Can you work these out from the model? Positions are in its coordinate system, mm. Face numbers are marked on the shaded views. A direction names the side the tool comes from. Give positions to 0.01 mm unless a question says otherwise; leave off trailing zeros. Loops run counter-clockwise (first coordinate to the right, second up) from the corner with the lowest first, then second, coordinate; pieces in that order, holes last. Notation, with made-up numbers: (-37.5, 34) -> (-15.5, 34) arc R14 cw to (-15.5, 52) -> close; hole circle Ø11 at (44.25, -33). An arc over 180 degrees is marked (long way). Return JSON: item names as keys, results as strings. Group by question number.
Q1. Thinking about a two-plate mould opening in Y: for the marked faces 1, 2 and 3, which applies, pulls with the +Y half, pulls with the -Y half, needs draft (parallel to the pull), parting line crosses it, or undercut?
Q2. I need wall thicknesses on line 1 along Z through (x, y) = (-3, 16.5); line 2 along Y through (x, z) = (-24, 3.75); line 3 along X through (y, z) = (14, 60). Which ranges of each line are inside material? Lowest first, please. Write a range as [from, to].
Q3. Will these pins go through, and if not, where does the flat tip stop? pin 1 (1.5 mm diameter, centred on x = -22, y = -9, fed in from +Z); pin 2 (12 mm diameter, centred on x = -5.5, z = 28, fed in from -Y); pin 3 (9 mm diameter, centred on x = -13.5, y = 3.5, fed in from +Z); pin 4 (11.5 mm diameter, centred on y = -3, z = 39, fed in from -X).
Q4. Suppose I cut it at A-A, the plane y = 14. Please give me the cut outline in (x, z).
Q5. Suppose I cut it at C-C, the plane x = 22.5. Please give me the cut outline in (y, z).
Q6. Suppose I cut it at B-B, the plane z = 51. Please give me the cut outline in (x, y).
Q7. Which directions (+Z, -Z, +X, -X, +Y, -Y) give clear straight access to the entire face, cutting with the end or side of a thin tool? Please do the marked faces 4, 5, 6, 7 and 8.
Q8. Suppose I cut it at D-D, the plane x = 12. Please give me the cut outline in (y, z).
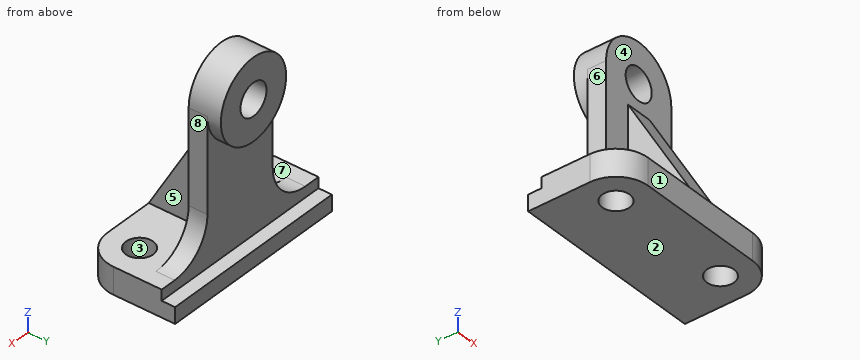
```python
from build123d import *

# Parameters (mm, degrees)
CROQUIS1_W              = 72
CROQUIS1_H              = 35
CROQUIS1_R              = 5.1
SALIENTE_EXTRUIR1_DEPTH = 10
REDONDEO1_R             = 12
CORTAR_EXTRUIR1_REACH   = 76.768
CROQUIS2_W              = 4
CROQUIS2_H              = 5
CROQUIS3_R              = 6
SALIENTE_EXTRUIR2_DEPTH = 7
SALIENTE_EXTRUIR4_START = 5
CROQUIS5_R              = 15
CROQUIS5_R_2            = 6
SALIENTE_EXTRUIR4_DEPTH = 5
REDONDEO2_R             = 15
NERVIO31_REACH          = 87.013
CROQUIS8_WALL_W         = 218.167556508
CROQUIS8_WALL_H         = 10


with BuildPart() as part:
    # Croquis1 → Saliente-Extruir1 (new body)
    with BuildSketch(Plane.XY):
        Rectangle(CROQUIS1_W, CROQUIS1_H)
        with Locations((-24, -5.5)):
            Circle(CROQUIS1_R, mode=Mode.SUBTRACT)
        with Locations((24, -5.5)):
            Circle(CROQUIS1_R, mode=Mode.SUBTRACT)
    extrude(amount=SALIENTE_EXTRUIR1_DEPTH)

    # Redondeo1
    redondeo1_edges = [part.edges().sort_by_distance(p)[0] for p in [
        (36, -17.5, 5),
        (-36, -17.5, 5),
    ]]
    fillet(redondeo1_edges, radius=REDONDEO1_R)

    # Croquis2 → Cortar-Extruir1 (cut, up to next)
    with BuildSketch(Plane.ZY.offset(36), mode=Mode.PRIVATE) as cortar_extruir1_sk1:
        with Locations((8, 15)):
            Rectangle(CROQUIS2_W, CROQUIS2_H)
    cortar_extruir1_tool1 = extrude(cortar_extruir1_sk1.sketch, amount=-CORTAR_EXTRUIR1_REACH, mode=Mode.PRIVATE) & part.part
    add(cortar_extruir1_tool1.solids().sort_by_distance((-36, 15, 8))[0], mode=Mode.SUBTRACT)

    # Croquis3 → Saliente-Extruir2 (add)
    with BuildSketch(Plane(origin=(0, 12.5, 0), x_dir=(1, 0, 0), z_dir=(0, 1, 0))):
        with BuildLine():
            Line((15, -60), (15, -10))
            Line((15, -10), (-15, -10))
            Line((-15, -10), (-15, -60))
            ThreePointArc((-15, -60), (0, -75), (15, -60))
        make_face()
        with Locations(Location((0, -60, 0), (0, 0, 270))):
            Circle(CROQUIS3_R, mode=Mode.SUBTRACT)
    extrude(amount=-SALIENTE_EXTRUIR2_DEPTH)

    # Croquis5 → Saliente-Extruir4 (add)
    with BuildSketch(Plane(origin=(0, 12.5, 0), x_dir=(1, 0, 0), z_dir=(0, 1, 0)).offset(SALIENTE_EXTRUIR4_START)):
        with Locations(Location((0, -60, 0), (0, 0, 270))):
            Circle(CROQUIS5_R)
        with Locations(Location((0, -60, 0), (0, 0, 270))):
            Circle(CROQUIS5_R_2, mode=Mode.SUBTRACT)
    extrude(amount=-SALIENTE_EXTRUIR4_DEPTH)

    # Redondeo2
    redondeo2_edges = [part.edges().sort_by_distance(p)[0] for p in [
        (-15, 9, 10),
        (15, 9, 10),
    ]]
    fillet(redondeo2_edges, radius=REDONDEO2_R)

    # Croquis8 wall → Nervio31 (add, up to next)
    with BuildSketch(Plane(origin=(0, -6, 30), x_dir=(0, 0.498471124258, 0.866906303058), z_dir=(0, -0.866906303058, 0.498471124258)), mode=Mode.PRIVATE) as nervio31_sk1:
        Rectangle(CROQUIS8_WALL_W, CROQUIS8_WALL_H)
    nervio31_tool1 = extrude(nervio31_sk1.sketch, amount=-NERVIO31_REACH, mode=Mode.PRIVATE) - part.part
    add(nervio31_tool1.solids().sort_by_distance((0, -6, 30))[0])


solid = part.part
```
Ans:
{
 "1": {"face 1": "pulls with the -Y half", "face 2": "needs draft", "face 3": "undercut"},
 "2": {"line 1": "z = [0, 6], [45.3, 54.8], [65.2, 74.7]", "line 2": "y = [-17.5, -10.6], [-0.4, 17.5]", "line 3": "x = [-15, -6], [6, 15]"},
 "3": {"pin 1": "passes through", "pin 2": "stops at y = -10.59", "pin 3": "stops at z = 71.63", "pin 4": "stops at x = -5"},
 "4": {"outline": "(-36, 0) -> (36, 0) -> (36, 6) -> (-36, 6) -> close; circle Ø30 at (0, 60); hole circle Ø12 at (0, 60)"},
 "5": {"outline": "(-17.5, 0) -> (-10.37, 0) -> (-10.37, 10) -> (-17.5, 10) -> close; (-0.63, 0) -> (17.5, 0) -> (17.5, 6) -> (12.5, 6) -> (12.5, 12.01) -> (5.5, 12.01) -> (5.5, 10) -> (-0.63, 10) -> close"},
 "6": {"outline": "(-15, 5.5) -> (15, 5.5) -> (15, 12.5) -> (12, 12.5) -> (12, 17.5) -> (-12, 17.5) -> (-12, 12.5) -> (-15, 12.5) -> close"},
 "7": {"face 4": "+Z, -Y", "face 5": "+Z, +X, -Y", "face 6": "+Z, -X, +Y, -Y", "face 7": "+Z, -X, -Y", "face 8": "+Z, +X, +Y, -Y"},
 "8": {"outline": "(-17.5, 0) -> (17.5, 0) -> (17.5, 6) -> (12.5, 6) -> (12.5, 51) -> (17.5, 51) -> (17.5, 69) -> (5.5, 69) -> (5.5, 10) -> (-17.5, 10) -> close"}
}
